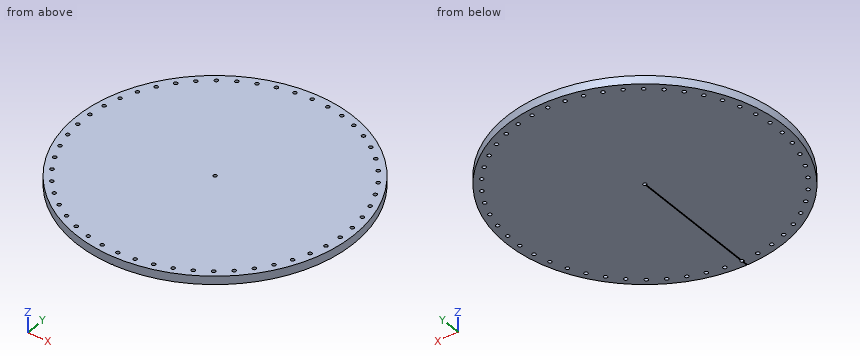
from build123d import *

# Parameters (mm, degrees)
SKETCH_R           = 300
SKETCH_R_2         = 4
PAD_DEPTH          = 18
SKETCH001_R        = 4
POCKET_DEPTH       = 1715.43907
POLARPATTERN_COUNT = 50
SKETCH002_W        = 2
SKETCH002_H        = 304.858551
POCKET001_DEPTH    = 2


with BuildPart() as part:
    # Sketch → Pad (new body)
    with BuildSketch(Plane.XY):
        Circle(SKETCH_R)
        Circle(SKETCH_R_2, mode=Mode.SUBTRACT)
    extrude(amount=PAD_DEPTH)

    # Sketch001 (on Face4 of Pad) → Pocket (cut, through all)
    with BuildSketch(Plane.XY.offset(18)):
        with Locations((0, 285)):
            Circle(SKETCH001_R)
    pocket = extrude(amount=-POCKET_DEPTH, mode=Mode.SUBTRACT)

    # PolarPattern: Pocket ×50 about axis
    polarpattern_axis = Axis((0, 0, 18), (0, 0, 1))
    for i in range(1, POLARPATTERN_COUNT):
        add(pocket.rotate(polarpattern_axis, i * 360 / POLARPATTERN_COUNT), mode=Mode.SUBTRACT)

    # Sketch002 (on Face2 of PolarPattern) → Pocket001 (cut)
    with BuildSketch(Plane(origin=(0, 0, 0), x_dir=(1, 0, 0), z_dir=(0, 0, -1))):
        with Locations((0, 152.429275)):
            Rectangle(SKETCH002_W, SKETCH002_H)
    extrude(amount=-POCKET001_DEPTH, mode=Mode.SUBTRACT)


solid = part.part
CAD build for the part. Positions are in the model's coordinates, mm. Coordinates: 2 decimals unless noted, no trailing zeros. Loops run counter-clockwise (first coordinate to the right, second up) from the corner with the lowest first, then second, coordinate; pieces in that order, holes last. Notation, with made-up numbers: (-34.5, 8) - (-2.5, 8) arc R29 ccw to (-2.5, 42) - close; hole circle Ø1 at (-35, 31.25). An arc over 180 degrees is marked (long way). Write item = value, one per line. Start each with the question number.
Q1. Flat gauge pins, fed straight in: pin 1 Ø3 at (y, z) = (-232.5, 4) entering from -X; pin 2 Ø7 at (x, y) = (-104.92, -264.99) entering from -Z; pin 3 Ø2 at (y, z) = (-15, 7) entering from -X; pin 4 Ø1.5 at (y, z) = (22.5, 6) entering from -X. Where does each tip first touch, or does it go through?
Q2. Cut at C-C, the plane x = 117.5. List the corners of the cut face in (y, z).
Q3. Cut at A-A, the plane y = -219. List the corners of the cut face in (x, z), then the cut area to 3 significant figures.
Q4. Cut at D-D, the plane x = -60. List the corners of the cut face in (y, z).
Q5. Drill centre lines: L1, parallel to X at y = 56.5, z = 8.25; L2, parallel to Y at x = 104.5, z = 13.5; L3, parallel to X at y = 85, z = 15.75. Where is each one in solid material? Low to high.
Q6. Cut at B-B, the plane z = 8. Give the number of separate pieces and of enclosed holes in the cut face, then the cut area to 3 significant figures.
Computed:
q1.pin_1 = -191.41
q1.pin_2 = through
q1.pin_3 = -299.67
q1.pin_4 = -299.21
q2.outline = (-276.03, 0) - (276.03, 0) - (276.03, 18) - (-276.03, 18) - close
q3.outline = (-205.03, 0) - (-1, 0) - (-1, 2) - (1, 2) - (1, 0) - (205.03, 0) - (205.03, 18) - (-205.03, 18) - close
q3.area = 7,380 mm²
q4.outline = (-293.94, 0) - (293.94, 0) - (293.94, 18) - (-293.94, 18) - close
q5.L1 = -294.63 to -282.48, -277.42 to 277.42, 282.48 to 294.63
q5.L2 = -281.21 to -268.96, -261.01 to 261.01, 268.96 to 281.21
q5.L3 = -287.71 to -273.62, -268.49 to 268.49, 273.62 to 287.71
q6.separate_pieces = 1
q6.enclosed_holes = 51
q6.area = 280,000 mm²
